Autodesk Inventor part; units mm, degrees
ref_plane "YZ Plane" through (0, 0, 0) normal (1, 0, 0) x (0, 1, 0)
ref_plane "XZ Plane" through (0, 0, 0) normal (0, 1, 0) x (-1, 0, 0)
ref_plane "XY Plane" through (0, 0, 0) normal (0, 0, 1) x (1, 0, 0)
sketch "Sketch1" plane through (0, 0, 0) normal (0, 1, 0) x (-1, 0, 0)
  line L0 (135.8628, 182.2707) -> (-199.1372, 182.2707)
  line L1 (-199.1372, 182.2707) -> (-199.1372, -117.7293)
  line L2 (-199.1372, -117.7293) -> (135.8628, -117.7293)
  line L3 (135.8628, -117.7293) -> (135.8628, 182.2707)
  circle A0 centre (-46.1372, -301.7293) radius 4.5
  circle A1 centre (19.8628, -367.7293) radius 4.5
  circle A2 centre (19.8628, -235.7293) radius 4.5
  circle A3 centre (85.8628, -301.7293) radius 4.5
  line L4 (83.3404, -354.6002) -> (128.9488, -400.2086)
  arc A4 (128.9488, -400.2086) -> (135.8628, -377.7293) centre (95.8628, -377.7293) ccw
  line L5 (135.8628, -377.7293) -> (135.8628, -117.7293)
  line L6 (135.8628, -117.7293) -> (-199.1372, -117.7293)
  line L7 (-199.1372, -117.7293) -> (-199.1372, -417.7293)
  line L8 (-199.1372, -417.7293) -> (95.8628, -417.7293)
  arc A5 (95.8628, -417.7293) -> (118.3422, -410.8152) centre (95.8628, -377.7293) ccw
  line L9 (118.3422, -410.8152) -> (72.7338, -365.2068)
  arc A6 (83.3404, -354.6002) -> (72.7338, -365.2068) centre (78.0371, -359.9035) ccw
  circle A7 centre (117.0128, -356.8793) radius 11.75
  circle A8 centre (75.0128, -398.8793) radius 11.75
  circle A9 centre (35.4128, -398.8793) radius 7.85
  circle A10 centre (117.0128, -317.2793) radius 7.85
  circle A11 centre (-180.2872, -136.5793) radius 7.85
  circle A12 centre (-180.2872, -398.8793) radius 7.85
  circle A13 centre (117.0128, -136.5793) radius 7.85
  point P0 (0, 0)
  point P1 (117.0128, 121.4207)
  point P2 (75.0128, 163.4207)
  point P3 (35.4128, 163.4207)
  point P4 (-180.2872, -98.8793)
  point P5 (-180.2872, 163.4207)
  point P6 (117.0128, 121.4207)
  point P7 (75.0128, 163.4207)
  point P8 (35.4128, 163.4207)
  point P9 (-180.2872, 163.4207)
  point P10 (-180.2872, -98.8793)
  dimension "d0" = 335
  dimension "d1" = 300
  dimension "d2" = 0
  dimension "d3" = 0
extrude "Extrusion1" add sketch "Sketch1" against normal blind 10.5 contours L3 L2 L1 L0
hole "Hole1" at (-117.0128, 0, 121.4207) at (-75.0128, 0, 163.4207) direction (0, -1, 0) diameter 12 end through all countersink diameter 23.5 countersink angle 90
hole "Hole2" at (-35.4128, 0, 163.4207) at (180.2872, 0, 163.4207) at (180.2872, 0, -98.8793) direction (0, -1, 0) diameter 8 end through all countersink diameter 15.7 countersink angle 90
fillet "Fillet1" radius 40 1 edges at (-135.8628, -5.25, 182.2707)
properties part number "Left bottom plate"
Geometry check sheet. Reference: the model listing, model coordinates, mm. Coordinates: 2 decimals unless noted, no trailing zeros. One line per item, written item: value. Start each with the question number.
(1) Scan lines: line 1 along X through (y, z) = (-1.25, 129); line 2 along X through (y, z) = (-5.25, -97); line 3 along Z through (x, y) = (-83, -1.5). Record each from-to range of solid material in increasing order. Write a range as [from, to].
(2) Release check for a two-part mould opening along Z. For faces 1 (the face through (34, -5, -117.729)), 2 (the face through (199.137, -5, 34)), 3 (the face through (181.819, -7.222, -95.184)) record: released by +Z, released by -Z, zero draft, split by the parting line, or undercut.
(3) Depth check by flat-ended pin: pin 1 (10.5 mm diameter, centred on x = 180.29, z = -98.88, fed in from +Y); pin 2 (19 mm diameter, centred on x = -117.01, z = 121.42, fed in from +Y); pin 3 (14 mm diameter, centred on x = -75.01, z = 163.42, fed in from +Y). Enter the tip coordinate at first touch or a pass-through.
Filled sheet:
1. line 1: [-135.86, -124.28], [-109.75, 199.14]
1. line 2: [-135.86, 176.76], [183.82, 199.14]
1. line 3: [-117.73, 157], [169.84, 182.27]
2. face 1: released by -Z
2. face 2: zero draft
2. face 3: undercut
3. pin 1: y = -2.6
3. pin 2: y = -2.25
3. pin 3: y = -4.75
